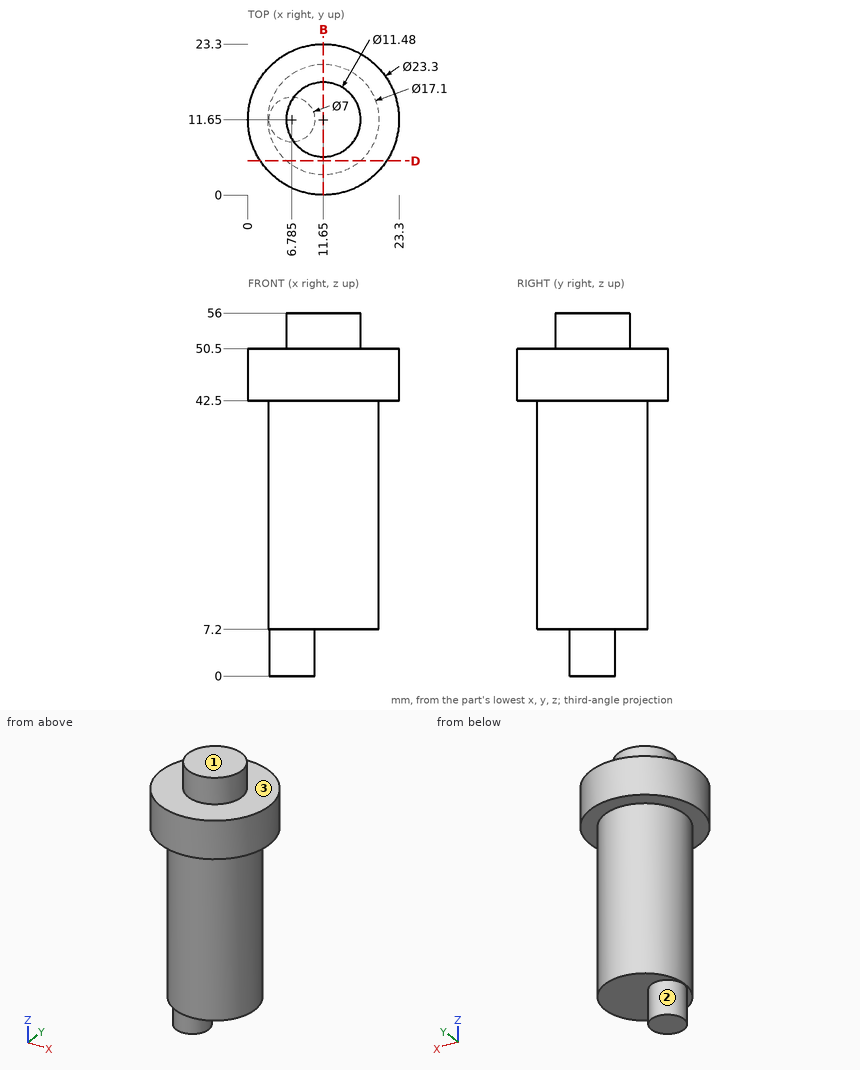
Design review of the part shown in the three views and the two pictorial views. Dimensions are in mm from the part's minimum x, y and z. A direction names the side the tool comes from. Coordinates: 2 decimals unless noted, no trailing zeros. Order: outer loops, then holes, each group sorted by start corner. A loop starts at its lowest first (then second) coordinate and runs counter-clockwise, first axis right, second up. Notation, with made-up numbers: (78.5, 68) -> (123.5, 68) arc R11 cw to (123.5, 84) -> close; hole circle Ø11 at (-30, 36.5). An arc over 180 degrees is marked (long way). Use one line per item in the form item = value. Start each with the question number.
(1) Add section B-B on x = 11.65. State the section outline as (y, z) points.
(2) For the marked faces 1, 2 and 3, list the 3-axis set-ups (+Z, -Z, +X, -X, +Y, -Y) from which the entire face can be reached by the end or side of a thin tool; tool diameter is ignored.
(3) Add section D-D on y = 5.25. State the section outline as (x, z) points (1 decimal), plus the area to 3 significant figures.
(4) Insertion check: pin 1 (1 mm diameter, centred on y = 7, z = 9, fed in from -X) (1 decimal); pin 2 (1 mm diameter, centred on x = 7.5, z = 20, fed in from +Y); pin 3 (8 mm diameter, centred on x = 10.5, z = 15.5, fed in from +Y). Each pin has a flat end and moves straight along its axis. Give the tip position at first contact, or say it passes through.
(5) For probe 1 along Z at (x, y) = (13.75, 12.5); probe 2 along Z at (x, y) = (19, 7.75); probe 3 along Y at (x, z) = (8.25, 19) (1 decimal), list the stretches that pass through material, from the lowest coordinate up.
Answer block:
q1.outline = (0, 42.5) -> (3.1, 42.5) -> (3.1, 7.2) -> (20.2, 7.2) -> (20.2, 42.5) -> (23.3, 42.5) -> (23.3, 50.5) -> (17.39, 50.5) -> (17.39, 56) -> (5.91, 56) -> (5.91, 50.5) -> (0, 50.5) -> close
q2.face_1 = +Z, +X, -X, +Y, -Y
q2.face_2 = -Z
q2.face_3 = +Z
q3.outline = (1.9, 42.5) -> (6, 42.5) -> (6, 7.2) -> (17.3, 7.2) -> (17.3, 42.5) -> (21.4, 42.5) -> (21.4, 50.5) -> (1.9, 50.5) -> close
q3.area = 556 mm²
q4.pin_1 = 4.2
q4.pin_2 = 19.38
q4.pin_3 = 20.2
q5.probe_1 = 7.2 to 56
q5.probe_2 = 7.2 to 50.5
q5.probe_3 = 3.8 to 19.5
